Input: part model. Units: mm. Frame: model coordinates. Face numbers are marked on the shaded views. A direction names the side the tool comes from. Give positions to 0.01 mm unless a question says otherwise; leave off trailing zeros. Order: outer loops, then holes, each group sorted by start corner. A loop starts at its lowest first (then second) coordinate and runs counter-clockwise, first axis right, second up. Notation, with made-up numbers: (67, 75) - (81, 75) arc R22 cw to (81, 89) - close; hole circle Ø2 at (5, 17.25). An arc over 180 degrees is marked (long way). Answer in a Markdown table with one row per item. Add a question column.
1. Section query D-D on y = 1.25. Return loops of the section in (x, z).
2. Section query A-A on x = 0. Return loops of the section in (y, z).
3. Section query B-B on z = -18.5. Return loops of the section in (x, y).
4. Access query for the marked faces 4 and 5. Directions: +Z, -Z, +X, -X, +Y, -Y. A direction counts if a zero-diameter tool reaches every point of the face in a straight line with its end or side. Return the directions, or none.
5. Ray query, line 1 (Z direction, x = 25, y = 1.5); line 2 (Y direction, x = 0, z = -33.25); line 3 (X direction, y = 7.25, z = -29). Return the intervals inside material, ascending. Write a range as [from, to].
6. Mould query, pull axis X, two halves, no side actions, for the marked faces 1, 2 and 3. Classes: released by +X, released by -X, zero draft, split by the parting line, or undercut.
7. Section query C-C on x = 19.5. Return loops of the section in (y, z), and give its area (3 significant figures).
Autodesk Inventor part; units mm, degrees
ref_plane "YZ Plane" through (0, 0, 0) normal (1, 0, 0) x (0, 1, 0)
ref_plane "XZ Plane" through (0, 0, 0) normal (0, 1, 0) x (-1, 0, 0)
ref_plane "XY Plane" through (0, 0, 0) normal (0, 0, 1) x (1, 0, 0)
sketch "Sketch1" plane through (0, 0, 0) normal (0, 1, 0) x (-1, 0, 0)
  line L0 (-30, 16.5) -> (30, 16.5)
  line L1 (32, 14.5) -> (32, -14.5)
  line L2 (-32, -14.5) -> (-32, 14.5)
  arc A0 (-32, -14.5) -> (-30, -16.5) centre (-30, -14.5) ccw
  arc A1 (-30, 16.5) -> (-32, 14.5) centre (-30, 14.5) ccw
  arc A2 (32, 14.5) -> (30, 16.5) centre (30, 14.5) ccw
  arc A3 (30, -16.5) -> (32, -14.5) centre (30, -14.5) ccw
  line L3 (-35, 14.5) -> (-35, -34.5)
  line L4 (35, -34.5) -> (35, 14.5)
  arc A4 (35, 14.5) -> (30, 19.5) centre (30, 14.5) ccw
  line L5 (30, 19.5) -> (-30, 19.5)
  arc A5 (-30, 19.5) -> (-35, 14.5) centre (-30, 14.5) ccw
  line L6 (35, -34.5) -> (-35, -34.5)
  line L7 (-22, -16.5) -> (-22, -19.5)
  line L8 (22, -16.5) -> (22, -19.5)
  line L9 (30, -16.5) -> (22, -16.5)
  line L10 (-22, -16.5) -> (-30, -16.5)
  line L11 (-30, -19.5) -> (-22, -19.5)
  line L12 (22, -19.5) -> (30, -19.5)
  line L13 (32, -31.5) -> (-32, -31.5)
  line L14 (-32, -31.5) -> (-32, -21.5)
  line L15 (-32, -14.5) -> (-32, 14.5)
  line L16 (32, 14.5) -> (32, -14.5)
  line L17 (32, -21.5) -> (32, -31.5)
  line L18 (-30, -19.5) -> (-32, -21.5)
  line L19 (32, -21.5) -> (30, -19.5)
  point P0 (0, 0)
  point P1 (32, -16.5)
  point P2 (32, 16.5)
  point P3 (-32, -16.5)
  point P4 (-32, -19.5)
  point P5 (32, -19.5)
  dimension "d0" = 64
  dimension "d1" = 33
  dimension "d2" = 32
  dimension "d3" = 16.5
  dimension "d4" = 2
  dimension "d5" = 3
  dimension "d6" = 70
  dimension "d9" = 10
  dimension "d10" = 10
  dimension "d11" = 20
  dimension "d12" = 3
  dimension "d13" = 2
  dimension "d14" = 2
  dimension "d15" = 2
  dimension "d16" = 2
extrude "Extrusion1" add sketch "Sketch1" along normal blind 10
sketch "Sketch2" plane through (35, 0, -34.5) normal (0, 0, -1) x (-1, 0, 0)
  line L0 (0, 10) -> (70, 0)
  line L1 (70, 10) -> (0, 0)
  circle A0 centre (35, 5) radius 1.75
  point P0 (35, 0)
  dimension "d19" = 3.5
extrude "Extrusion2" cut sketch "Sketch2" against normal blind 10
equation "\"BendRadius\" = Thickness"
equation "\"BendReliefWidth\" = Thickness"
equation "\"BendReliefDepth\" = 0.5 * Thickness"
equation "\"CornerReliefSize\" = 4 * Thickness"
equation "\"MinimumRemnant\" = 2 * Thickness"
equation "\"TransitionRadius\" = BendRadius"
equation "\"JacobiRadiusSize\" = BendRadius"
equation "\"GapSize\" = Thickness"
properties part number "dcdcSupport"
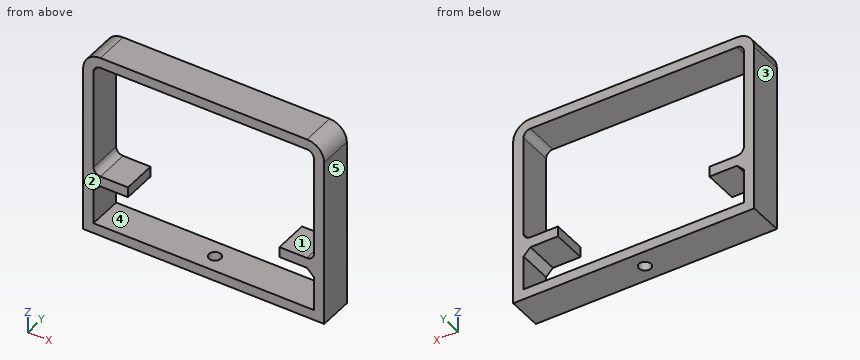
Answer:
| question | item | result |
|---|---|---|
| 1 | outline | (-35, -34.5) - (35, -34.5) - (35, 14.5) arc R5 ccw to (30, 19.5) - (-30, 19.5) arc R5 ccw to (-35, 14.5) - close; hole (-32, -31.5) - (32, -31.5) - (32, -21.5) - (30, -19.5) - (22, -19.5) - (22, -16.5) - (30, -16.5) arc R2 ccw to (32, -14.5) - (32, 14.5) arc R2 ccw to (30, 16.5) - (-30, 16.5) arc R2 ccw to (-32, 14.5) - (-32, -14.5) arc R2 ccw to (-30, -16.5) - (-22, -16.5) - (-22, -19.5) - (-30, -19.5) - (-32, -21.5) - close |
| 2 | outline | (0, -34.5) - (3.25, -34.5) - (3.25, -31.5) - (0, -31.5) - close; (0, 16.5) - (10, 16.5) - (10, 19.5) - (0, 19.5) - close; (6.75, -34.5) - (10, -34.5) - (10, -31.5) - (6.75, -31.5) - close |
| 3 | outline | (-35, 0) - (-22, 0) - (-22, 10) - (-35, 10) - close; (22, 0) - (35, 0) - (35, 10) - (22, 10) - close |
| 4 | face 4 | +Y, -Y |
| 4 | face 5 | +Z, -Z, +X, +Y, -Y |
| 5 | line 1 | z = [-34.5, -31.5], [-19.5, -16.5], [16.5, 19.5] |
| 5 | line 2 | y = [0, 3.25], [6.75, 10] |
| 5 | line 3 | x = [-35, -32], [32, 35] |
| 6 | face 1 | undercut |
| 6 | face 2 | zero draft |
| 6 | face 3 | released by -X |
| 7 | outline | (0, -34.5) - (10, -34.5) - (10, -31.5) - (0, -31.5) - close; (0, 16.5) - (10, 16.5) - (10, 19.5) - (0, 19.5) - close |
| 7 | area | 60.0 mm² |
